from build123d import *

# Parameters (mm, degrees)
F1_DEPTH    = 2.7
F2_T1_DEPTH = 2.7
F3_R        = 9.99999
F5_DEPTH    = 1.2


# Not quite as in the source:
# - a fillet or chamfer that OpenCascade refuses, or shapes differently, is made with other operations: its cross-section is extruded or revolved along the edge and cut away or added
# - a fillet or chamfer is up to 0.001 mm smaller than in the source, because OpenCascade refuses the exact size


with BuildPart() as f1:
    # F0 (on Top) → F1 (new body)
    with BuildSketch(Plane.XY):
        Polygon((-10, 0), (-3.6, 0), (-3.6, 13.4), (0, 13.4), (3.6, 13.4), (3.6, 0), (10, 0), (10, 25), (0, 25), (-10, 25), align=None)
    extrude(amount=F1_DEPTH)

    # F2: fillet of radius 4 on 2 edges, made by hand

    # F2_s2 → F2_t1 (join)
    with BuildSketch(Plane.XY):
        with BuildLine():
            ThreePointArc((0.4, 13.4), (-2.4284271247, 12.2284271247), (-3.6, 9.4))
            Line((-3.6, 9.4), (-3.6, 13.4))
            Line((-3.6, 13.4), (0.4, 13.4))
        make_face()
        with BuildLine():
            ThreePointArc((3.6, 9.4), (2.4284271247, 12.2284271247), (-0.4, 13.4))
            Line((-0.4, 13.4), (3.6, 13.4))
            Line((3.6, 13.4), (3.6, 9.4))
        make_face()
    extrude(amount=F2_T1_DEPTH)

    # F3 (radius 10 in the source; OpenCascade refuses exactly that, so slightly less here)
    f3_edges = [f1.edges().sort_by_distance(p)[0] for p in [
        (-10, 25, 1.35),
        (10, 25, 1.35),
    ]]
    fillet(f3_edges, radius=F3_R)

    # F4 (on Top) → F5 (cut)
    with BuildSketch(Plane.XY):
        with BuildLine():
            Line((-11.2521313131, -1.0476741055), (-5, -1.0476741055))
            Line((-5, -1.0476741055), (-5, 10))
            ThreePointArc((-5, 10), (-3.5355339059, 13.5355339059), (0, 15))
            ThreePointArc((0, 15), (3.5355339059, 13.5355339059), (5, 10))
            Line((5, 10), (5, -1.0476741055))
            Line((5, -1.0476741055), (11.2521313131, -1.0476741055))
            Line((11.2521313131, -1.0476741055), (11.2521313131, 27.1253902465))
            Line((11.2521313131, 27.1253902465), (0, 27.1253902465))
            Line((0, 27.1253902465), (-11.2521313131, 27.1253902465))
            Line((-11.2521313131, 27.1253902465), (-11.2521313131, -1.0476741055))
        make_face()
    extrude(amount=F5_DEPTH, mode=Mode.SUBTRACT)


solid = f1.part
Source: CAD feature listing. Evaluate the final solid. Frame: model axes, mm. A direction names the side the tool comes from. Round coordinates to 2 decimals unless told otherwise and drop trailing zeros. Order: outer loops, then holes, each group sorted by start corner. A loop starts at its lowest first (then second) coordinate and runs counter-clockwise, first axis right, second up. Notation, with made-up numbers: (89.5, 53.25) - (132.5, 53.25) arc R21 cw to (132.5, 81.25) - close; hole circle Ø9 at (87, -24.75). An arc over 180 degrees is marked (long way). Use a Markdown table: item, result. Add a question column.
1. Section query A-A (y = 5.5). Return the cut outline in (x, z), then the cut area to 3 significant figures.
2. Line query: probe 1 along X at (y, z) = (4.75, 2.6); probe 2 along Z at (x, y) = (-4.75, 16.25); probe 3 along X at (y, z) = (5.5, 1). Output: solid intervals per line, ascending.
3. Section query C-C (x = -1.25). Return the cut outline in (y, z).
4. Section query D-D (y = 21). Return the cut outline in (x, z), then the cut area to 3 significant figures.
5. Mould query, pull axis X, two halves, no side actions, for faces 1 (the flat face through (5, 5, 1)), 2 (the cylindrical face through (2.594, 12.053, 1.331)), 3 (the cylindrical face through (-6.99, 22.15, 1.96)). Classes: +X half, -X half, draft (parallel to the pull), parting line (faces both ways), or undercut.
6. Set-up query: faces 4 (the flat face through (-0.1, 15.5, 1.2)), 5 (the flat face through (-6, 0, 2)), 6 (the flat face through (-5, 5, 1)), 7 (the cylindrical face through (7.15, 21.99, 1.96)), 8 (the cylindrical face through (-2.54, 12.11, 1.33)). Return all of +Z, -Z, +X, -X, +Y, -Y with unobstructed straight access to the full face (end or side cutting, diameter ignored); none if empty.
7. First-contact query: pin 1 (1.5 mm diameter, centred on y = 16, z = 1, fed in from -X); pin 2 (0.6 mm diameter, centred on y = 4, z = 0.5, fed in from -X); pin 3 (1.5 mm diameter, centred on x = 2.5, y = 22.5, fed in from -Z). Flat tips, straight axial feed; report the tip coordinate or a pass-through.
8. Section query B-B (z = 0.85). Return the cut outline in (x, y).
Derived:
| question | item | result |
|---|---|---|
| 1 | outline | (-10, 1.2) - (-5, 1.2) - (-5, 0) - (-3.6, 0) - (-3.6, 2.7) - (-10, 2.7) - close; (3.6, 0) - (5, 0) - (5, 1.2) - (10, 1.2) - (10, 2.7) - (3.6, 2.7) - close |
| 1 | area | 22.6 mm2 |
| 2 | probe 1 | -10 to -3.6, 3.6 to 10 |
| 2 | probe 2 | 1.2 to 2.7 |
| 2 | probe 3 | -5 to -3.6, 3.6 to 5 |
| 3 | outline | (13.04, 0) - (14.84, 0) - (14.84, 1.2) - (24.92, 1.2) - (24.92, 2.7) - (13.04, 2.7) - close |
| 4 | outline | (-8, 1.2) - (8, 1.2) - (8, 2.7) - (-8, 2.7) - close |
| 4 | area | 24.0 mm2 |
| 5 | face 1 | +X half |
| 5 | face 2 | undercut |
| 5 | face 3 | -X half |
| 6 | face 4 | -Z, +Y |
| 6 | face 5 | +Z, -Z, +X, -X, -Y |
| 6 | face 6 | -Z, -X, +Y, -Y |
| 6 | face 7 | +Z, -Z, +X, +Y |
| 6 | face 8 | +Z, -Z, -Y |
| 7 | pin 1 | x = -10 |
| 7 | pin 2 | x = -5 |
| 7 | pin 3 | z = 1.2 |
| 8 | outline | (-5, 0) - (-3.6, 0) - (-3.6, 9.4) arc R4 cw to (0, 13.38) arc R4 cw to (3.6, 9.4) - (3.6, 0) - (5, 0) - (5, 10) arc R5 ccw to (-5, 10) - close |
